Autodesk Inventor part; units mm, degrees
ref_plane "Work Plane1" through (0, 0, 0) normal (0, -1, 0) x (1, 0, 0)
ref_plane "YZ Plane" through (0, 0, 0) normal (1, 0, 0) x (0, 1, 0)
ref_plane "XZ Plane" through (0, 0, 0) normal (0, 1, 0) x (-1, 0, 0)
sketch "Эскиз1" plane through (0, 0, 0) normal (1, 0, 0) x (0, 1, 0)
  circle A0 centre (0, 0) radius 10.25
  circle A1 centre (0, 0) radius 6.5
  dimension "d0" = 20.5
  dimension "d1" = 13
extrude "Базовый элемент" add sketch "Эскиз1" along normal blind 1
sketch "Эскиз2" plane through (1, 0, 0) normal (1, 0, 0) x (0, 0, -1)
  circle A0 centre (0, 0) radius 10.25
  line L0 (0, 0) -> (0, 10.25) construction
  arc A1 (1.6035, 10.1238) -> (-1.6035, 10.1238) centre (0, 0) ccw
  arc A2 (1.3101, 8.2719) -> (-1.3101, 8.2719) centre (0, 0) ccw
  line L1 (-1.3101, 8.2719) -> (-1.6035, 10.1238)
  line L2 (1.3101, 8.2719) -> (1.6035, 10.1238)
  line L3 (-1.3101, 8.2719) -> (0, 0) construction
  line L4 (0, 0) -> (1.3101, 8.2719) construction
  dimension "d4" = 18
  dimension "d5" = 16.75
extrude "Вырез" cut sketch "Эскиз2" against normal through all contours L2 A2 L1 A0 picked at (0.1461, 9.6118)
fillet "Сопряжение1" radius 0.3075 2 edges at (0.5, 8.2719, 1.3101) (0.5, 8.2719, -1.3101)
pattern_circular "Вырезы" count 10 over 360 about axis through (0, 0, 0) along (1, 0, 0) of "Вырез", "Сопряжение1"
ref_plane "Work Plane1" through (0, 0, 0) normal (0, -1, 0) x (1, 0, 0)
equation "\"d0\" = SD2"
equation "\"d1\" = SD1"
equation "\"d2\" = SD"
equation "\"d5\" = 0.5 * SD2 + 0.5 * SD1"
equation "\"d6\" = SD"
equation "\"d8\" = 0.015 * SD2"
equation "\"SD\" = 1"
equation "\"SD1\" = 13"
equation "\"SD2\" = 20.5"
equation "\"NND\" = 12"
properties part number "DIN 6797 - A 13" material "Сталь, мягкая"
Build history of the part. All positions in model axes, mm. A direction names the side the tool comes from. Round coordinates to 2 decimals unless told otherwise and drop trailing zeros. Write each loop counter-clockwise with the first axis right and the second up, starting at its lowest first coordinate (ties: lowest second). Pieces come first, ordered by that corner, then holes.
1) 3-axis set-ups, long thin cutter, end or side, ignore diameter. For faces 4 (the flat face through (0.51, 8.42, 4.29)), 5 (the flat face through (0.5, -6.7, -6.7)), 6 (the cylindrical face through (0.507, 6.784, 4.911)), 7 (the flat face through (0.51, 8.42, -4.29)), 8 (the flat face through (0, -5, 5)): which of +Z, -Z, +X, -X, +Y, -Y reach the whole face in a straight line?
2) Drill centre lines: probe 1 along Y at (x, z) = (0.65, 9); probe 2 along Z at (x, y) = (0.2, 0); probe 3 along Z at (x, y) = (0.1, 7). Where is each one in solid material? Low to high.
3) Mould opens along Y. For faces 1 (the cylindrical face through (0.493, -9.755, 3.146)), 2 (the cylindrical face through (0.507, -6.784, -4.911)), 3 (the flat face through (0.5, 6.7, 6.7)) say: +Y half, -Y half, draft (parallel to the pull), parting line (faces both ways), or undercut.
4) Band-saw the part on A-A, the plane z = 0. List the corners of the cut face in (x, y) (3 decimals).
5) Band-saw the part on C-C, the plane y = -7. List the corners of the cut face in (x, z).
6) Band-saw the part on B-B, the plane y = 0. List the corners of the cut face in (x, z).
Ans:
1. face 4: +Z, +X, -X
1. face 5: +X, -X, -Y
1. face 6: +X, -X
1. face 7: -Z, +X, -X
1. face 8: +Z, -Z, -X, +Y, -Y
2. probe 1: y = -4.91 to -4.59, -1.43 to 1.43, 4.59 to 4.91
2. probe 2: z = -10.25 to -6.5, 6.5 to 10.25
2. probe 3: z = -7.49 to -7, -4.6 to 4.6, 7 to 7.49
3. face 1: -Y half
3. face 2: undercut
3. face 3: +Y half
4. outline: (0, -8.375) - (1, -8.375) - (1, -6.5) - (0, -6.5) - close; (0, 6.5) - (1, 6.5) - (1, 8.375) - (0, 8.375) - close
5. outline: (0, -7.49) - (1, -7.49) - (1, -7) - (0, -7) - close; (0, -4.6) - (1, -4.6) - (1, 4.6) - (0, 4.6) - close; (0, 7) - (1, 7) - (1, 7.49) - (0, 7.49) - close
6. outline: (0, -10.25) - (1, -10.25) - (1, -6.5) - (0, -6.5) - close; (0, 6.5) - (1, 6.5) - (1, 10.25) - (0, 10.25) - close
